```python
from build123d import *

# Parameters (mm, degrees)
BOSS_EXTRUDE1_DEPTH      = 1.5
BOSS_EXTRUDE1_DEPTH_BACK = 1.5
BOSS_EXTRUDE2_DEPTH      = 234
FILLET1_R                = 37
FILLET2_R                = 37
FILLET3_R                = 18
FILLET4_R                = 18


with BuildPart() as part:
    # Sketch1 → Boss-Extrude1 (new, two sides: drawn at the far end of the back side and taken through both)
    with BuildSketch(Plane.XY.offset(-BOSS_EXTRUDE1_DEPTH_BACK)):
        Polygon((0, 0), (0, 234), (184, 49), (218, -80), align=None)
    extrude(amount=BOSS_EXTRUDE1_DEPTH + BOSS_EXTRUDE1_DEPTH_BACK)

    # Sketch3 → Boss-Extrude2 (add)
    with BuildSketch(Plane(origin=(0, 0, 0), x_dir=(1, 0, 0), z_dir=(0, 1, 0))):
        with BuildLine():
            Line((0, 0), (0, 20))
            Line((0, 20), (-4.431457505, 20))
            ThreePointArc((-4.431457505, 20), (-1, 0), (-4.431457505, -20))
            Line((-4.431457505, -20), (0, -20))
            Line((0, -20), (0, 0))
        make_face()
    extrude(amount=BOSS_EXTRUDE2_DEPTH)

    # Fillet1
    # the kernel refuses this fillet: 37 mm, written as the material it takes off along each edge
    with BuildSketch(Plane(origin=(0, -43.895475262, -20), x_dir=(-1, 0, 0), z_dir=(0, 1, 0))) as fillet1_piece_1:
        with BuildLine():
            CenterArc((37, 17.558190105), FILLET1_R, 180, 28.329773325)
            Line((0, 17.558190105), (-0.74, 17.558190105))
            Line((-0.74, 17.558190105), (-0.74, 0))
            Line((-0.74, 0), (0, -0.74))
            ThreePointArc((0, -0.74), (2.215728753, -0.74), (3.780086655, -0.351163802))
            Line((3.780086655, -0.351163802), (4.431457505, 0))
        make_face()
    extrude(amount=321.790950524, mode=Mode.SUBTRACT)

    # Fillet2
    # the kernel refuses this fillet: 37 mm, written as the material it takes off along each edge
    with BuildSketch(Plane(origin=(0, -43.895475262, 20), x_dir=(-1, 0, 0), z_dir=(0, 1, 0))) as fillet2_piece_1:
        with BuildLine():
            CenterArc((37, -17.558190105), FILLET2_R, 151.670226675, 28.329773325)
            Line((0, -17.558190105), (-0.74, -17.558190105))
            Line((-0.74, -17.558190105), (-0.74, 0))
            Line((-0.74, 0), (0, 0.74))
            ThreePointArc((0, 0.74), (2.215728753, 0.74), (3.780086655, 0.351163802))
            Line((3.780086655, 0.351163802), (4.431457505, 0))
        make_face()
    extrude(amount=321.790950524, mode=Mode.SUBTRACT)

    # Fillet3
    # the kernel refuses this fillet: 18 mm, written as the material it adds along each edge
    with BuildSketch(Plane(origin=(0, -38.219598529, 1.5), x_dir=(-0.1453745067000553, 0, 0.9893766991402797), z_dir=(0, 1, 0))) as fillet3_piece_1_section:
        with BuildLine():
            CenterArc((15.586318472, 17.742173215), FILLET3_R, 188.358966638, 71.931795215)
            Line((-2.222462113, 15.125432094), (-4.003340171, 14.863757982))
            Line((-4.003340171, 14.863757982), (-1.780878058, -0.261674112))
            Line((-1.780878058, -0.261674112), (0.261674112, -1.780878058))
            ThreePointArc((0.261674112, -1.780878058), (1.193478877, -1.64396291), (12.247081967, -1.774217321))
            Line((12.247081967, -1.774217321), (12.550648922, 0))
        make_face()
    fillet3_piece_1 = extrude(amount=272.219598529, mode=Mode.PRIVATE)
    fillet3_piece_1 = fillet3_piece_1 - Plane(origin=(-61, -0.93503603, 0), x_dir=(0.9428090415820632, 0, -0.3333333333333337), z_dir=(0, -1, 0)) * Cylinder(60, 605, mode=Mode.PRIVATE)
    fillet3_piece_1 = split(fillet3_piece_1, bisect_by=Plane(origin=(6.052795765, -2.221209455, 3.73592086), z_dir=(0.34450770303612605, 0.9387834907734437, 0)), keep=Keep.TOP, mode=Mode.PRIVATE)
    fillet3_piece_1 = split(fillet3_piece_1, bisect_by=Plane(origin=(120.710503396, 112.633461259, 3.73592086), z_dir=(-0.7090204561204898, -0.7051879131144355, 0)), keep=Keep.TOP, mode=Mode.PRIVATE)
    add(fillet3_piece_1)
    with BuildSketch(Plane(origin=(0, 0, 1.5), x_dir=(-0.14537450670005528, 0, 0.9893766991402797), z_dir=(0, 1, 0))) as fillet3_piece_2_section:
        with BuildLine():
            CenterArc((15.586318472, 17.742173215), FILLET3_R, 188.358966638, 71.931795215)
            Line((-2.222462113, 15.125432094), (-4.003340171, 14.863757982))
            Line((-4.003340171, 14.863757982), (-1.780878058, -0.261674112))
            Line((-1.780878058, -0.261674112), (0.261674112, -1.780878058))
            ThreePointArc((0.261674112, -1.780878058), (1.193478877, -1.64396291), (12.247081967, -1.774217321))
            Line((12.247081967, -1.774217321), (12.550648922, 0))
        make_face()
    fillet3_piece_2 = extrude(amount=272.219598529, mode=Mode.PRIVATE)
    fillet3_piece_2 = fillet3_piece_2 - Plane(origin=(-61, 0.334778788, 0), x_dir=(0.9428090415820632, 0, -0.3333333333333337), z_dir=(0, -1, 0)) * Cylinder(60, 605, mode=Mode.PRIVATE)
    fillet3_piece_2 = split(fillet3_piece_2, bisect_by=Plane(origin=(-1.045097549, 0.383522036, 11.887652285), z_dir=(-0.34450770303612605, -0.9387834907734437, 0)), keep=Keep.TOP, mode=Mode.PRIVATE)
    add(fillet3_piece_2)

    # Fillet4
    # the kernel refuses this fillet: 18 mm, written as the material it adds along each edge
    with BuildSketch(Plane(origin=(0, -38.219598529, -1.5), x_dir=(-0.14537450670005567, 0, -0.9893766991402797), z_dir=(0, 1, 0))) as fillet4_piece_1_section:
        with BuildLine():
            CenterArc((15.586318472, -17.742173215), FILLET4_R, 99.709238147, 71.931795215)
            Line((-2.222462113, -15.125432094), (-4.003340171, -14.863757982))
            Line((-4.003340171, -14.863757982), (-1.780878058, 0.261674112))
            Line((-1.780878058, 0.261674112), (0.261674112, 1.780878058))
            ThreePointArc((0.261674112, 1.780878058), (1.193478877, 1.64396291), (12.247081967, 1.774217321))
            Line((12.247081967, 1.774217321), (12.550648922, 0))
        make_face()
    fillet4_piece_1 = extrude(amount=272.219598529, mode=Mode.PRIVATE)
    fillet4_piece_1 = fillet4_piece_1 - Plane(origin=(-61, -0.93503603, 0), x_dir=(0.9428090415820632, 0, -0.3333333333333337), z_dir=(0, -1, 0)) * Cylinder(60, 605, mode=Mode.PRIVATE)
    fillet4_piece_1 = split(fillet4_piece_1, bisect_by=Plane(origin=(120.710503396, 112.633461259, -3.73592086), z_dir=(-0.709020456120464, -0.7051879131144615, 0)), keep=Keep.TOP, mode=Mode.PRIVATE)
    fillet4_piece_1 = split(fillet4_piece_1, bisect_by=Plane(origin=(6.052795765, -2.221209455, -3.73592086), z_dir=(0.34450770303615846, 0.9387834907734318, 0)), keep=Keep.TOP, mode=Mode.PRIVATE)
    add(fillet4_piece_1)
    with BuildSketch(Plane(origin=(0, 0, -1.5), x_dir=(-0.1453745067000557, 0, -0.9893766991402797), z_dir=(0, 1, 0))) as fillet4_piece_2_section:
        with BuildLine():
            CenterArc((15.586318472, -17.742173215), FILLET4_R, 99.709238147, 71.931795215)
            Line((-2.222462113, -15.125432094), (-4.003340171, -14.863757982))
            Line((-4.003340171, -14.863757982), (-1.780878058, 0.261674112))
            Line((-1.780878058, 0.261674112), (0.261674112, 1.780878058))
            ThreePointArc((0.261674112, 1.780878058), (1.193478877, 1.64396291), (12.247081967, 1.774217321))
            Line((12.247081967, 1.774217321), (12.550648922, 0))
        make_face()
    fillet4_piece_2 = extrude(amount=272.219598529, mode=Mode.PRIVATE)
    fillet4_piece_2 = fillet4_piece_2 - Plane(origin=(-61, 0.334778788, 0), x_dir=(0.9428090415820632, 0, -0.3333333333333337), z_dir=(0, -1, 0)) * Cylinder(60, 605, mode=Mode.PRIVATE)
    fillet4_piece_2 = split(fillet4_piece_2, bisect_by=Plane(origin=(-1.045097549, 0.383522036, -11.887652285), z_dir=(-0.34450770303615846, -0.9387834907734318, 0)), keep=Keep.TOP, mode=Mode.PRIVATE)
    add(fillet4_piece_2)


solid = part.part
```
Could you check a few things on this model? Use its own coordinates, in mm. A direction names the side the tool comes from. Coordinates: 2 decimals unless noted, no trailing zeros. Write each loop counter-clockwise with the first axis right and the second up, starting at its lowest first coordinate (ties: lowest second). Pieces come first, ordered by that corner, then holes. Notation, with made-up numbers: M -36,31.5 L 8,31.5 A14 ccw 8,46.5 Z; hole C 51,-8.75 d7. An arc over 180 degrees is marked long. Answer as CSV lines item,"result". Start each with the question number.
1) I want a section at C-C, the plane x = 30. Please give me the cut outline in (y, z).
2) We'd pull the mould along Z, two halves only. Please class faces 1 (the cylindrical face through (-2.97, 115.36, -16.97)), 2 (the flat face through (100.42, -36.85, 0.69)), 3 (the cylindrical face through (-1, 115, 0)): +Z half, -Z half, draft (parallel to the pull), parting line (faces both ways), or undercut.
3) I want a section at D-D, the plane y = 32.5. Please give me the cut outline in (x, z), and give its area (3 significant figures).
4) For faces 4 (the flat face through (77.941, 155.635, 0.047)), 5 (the flat face through (96, 38, -1.5)), 6 (the flat face through (96, 38, 1.5)), which set-ups out of +Z, -Z, +X, -X, +Y, -Y let a thin tool reach every point of the face, with its end or its side?
5) For P1, Ø1, axis at x = 124.5, z = 0.5, coming from the -Y side; P2, Ø6, axis at y = 190, z = -13.5, coming from the +X side; P3, Ø5, axis at x = -1.5, z = -9.5, coming from the -Y side, each with a flat end and sliding along its axis, tell me the tip position at first contact or that it passes through.
6) Please list where these lines run through material, in increasing order: line 1 (Z direction, x = 130.5, y = 80); line 2 (X direction, y = 212, z = -11.5); line 3 (X direction, y = 12, z = 5). Write a range as from..to.
7) I want a section at A-A, the plane y = 67.5. Please give me the cut outline in (x, z).
8) I want a section at B-B, the plane z = -6.5. Please give me the cut outline in (x, y).
Data:
1,outline,"M -11.01,-1.5 L 203.84,-1.5 L 203.84,1.5 L -11.01,1.5 Z"
2,face 1,"-Z half"
2,face 2,"draft"
2,face 3,"undercut"
3,outline,"M -4.43,-20 A37 ccw -1.82,-13.92 A18 cw 15.29,-1.5 L 188.35,-1.5 L 188.35,1.5 L 15.29,1.5 A18 cw -1.82,13.92 A37 ccw -4.43,20 A60 cw Z"
3,area,"682 mm^2"
4,face 4,"+Z, -Z, +X, +Y"
4,face 5,"-Z, +X, +Y, -Y"
4,face 6,"+Z, +X, +Y, -Y"
5,P1,"stops at y = -45.87"
5,P2,"stops at x = -0.3"
5,P3,"stops at y = -0.32"
6,line 1,"z = -1.5..1.5"
6,line 2,"x = -2.11..-0.84"
6,line 3,"x = -1.21..4.62"
7,outline,"M -4.43,-20 A37 ccw -1.82,-13.92 A18 cw 15.29,-1.5 L 165.6,-1.5 L 165.6,1.5 L 15.29,1.5 A18 cw -1.82,13.92 A37 ccw -4.43,20 A60 cw Z"
8,outline,"M -1.35,0 L 0,0 L 2.84,-1.04 L 2.84,231.15 L 0,234 L -1.35,234 Z"
